```python
from build123d import *


with BuildPart() as part:
    # Çizim1 → Döndür1 (revolve)
    with BuildSketch(Plane.XY):
        Polygon((-235, 0), (235, 0), (235, 7.5), (227.5, 7.5), (227.5, 9), (-227.5, 9), (-227.5, 7.5), (-235, 7.5), align=None)
    revolve(axis=Axis((-235, 0, 0), (1, 0, 0)))

    # Çizim3 → M8 Dişli Delik1 (revolve, cut)
    with BuildSketch(Plane(origin=(235, 0, 0), x_dir=(0, 0, -1), z_dir=(0, 1, 0))):
        Polygon((0, 0), (0, 22.042926105), (3.4, 20), (3.4, 0), align=None)
    m8_di_li_delik1 = revolve(axis=Axis((241.35, 0, 0), (-1, 0, 0)), mode=Mode.SUBTRACT)

    # Aynalama1: M8 Dişli Delik1 across plane
    add(m8_di_li_delik1.mirror(Plane(origin=(0, 0, 0), x_dir=(0, 0, 1), z_dir=(1, 0, 0))), mode=Mode.SUBTRACT)


solid = part.part
```
Here's how the part is built. I have some questions about the finished solid (model axes, mm). A direction names the side the tool comes from. Coordinates: 2 decimals unless noted, no trailing zeros. Order: outer loops, then holes, each group sorted by start corner. A loop starts at its lowest first (then second) coordinate and runs counter-clockwise, first axis right, second up. Notation, with made-up numbers: (0.25, 85.25) -> (58.25, 85.25) arc R16 cw to (58.25, 113.25) -> close; hole circle Ø8 at (50.5, 86.5). An arc over 180 degrees is marked (long way). Return JSON: item names as keys, results as strings.
1) On a 3-axis mill with a long thin cutter (end or side, diameter ignored), from which of +Z, -Z, +X, -X, +Y, -Y can I reach the whole of each face in a straight line? I mean faces 1 (the flat face through (227.5, 2, 7.4)), 2 (the flat face through (-227.5, -2, 7.4)), 3 (the cylindrical face through (-3.185, -1.172, 8.923)). Say none if no direction works.
Conclusion:
{"face 1": "+X", "face 2": "-X", "face 3": "+X, -X"}
2) If I drill on probe 1 along Z at (x, y) = (-224, 0); probe 2 along Z at (x, y) = (228.25, 0); probe 3 along Y at (x, z) = (-9, -5), over which ranges is the centre line in solid material (lowest first)?
Conclusion:
{"probe 1": "z = -9 to -3.4, 3.4 to 9", "probe 2": "z = -7.5 to -3.4, 3.4 to 7.5", "probe 3": "y = -7.48 to 7.48"}
3) I'm going to push flat-ended pins straight in: P1, Ø2, axis at x = 152.5, z = -2, coming from the +Y side; P2, Ø4, axis at x = 100.5, y = -6, coming from the -Z side; P3, Ø6, axis at y = 0, z = 0, coming from the +X side. Where does each tip first touch, or does it pass through?
Conclusion:
{"P1": "stops at y = 8.94", "P2": "stops at z = -8.06", "P3": "stops at x = 214.76"}
4) If we section it at A-A on x = 59: List the corners of the cut face in (y, z) for me.
Conclusion:
{"outline": "circle Ø18 at (0, 0)"}
